from build123d import *

# Parameters (mm, degrees)
SKETCH1_R           = 1.55
SKETCH1_R_2         = 1.6
SKETCH1_W           = 15
SKETCH1_H           = 15
SKETCH1_W_2         = 52
SKETCH1_H_2         = 2.6
BOSS_EXTRUDE1_DEPTH = 2.5
SKETCH2_W           = 144
SKETCH2_H           = 40
BOSS_EXTRUDE2_DEPTH = 2.5


with BuildPart() as part:
    # Sketch1 → Boss-Extrude1 (new body)
    with BuildSketch(Plane(origin=(0, 0, 0), x_dir=(1, 0, 0), z_dir=(0, 1, 0))):
        Polygon((-72, -25), (-76, -25), (-76, 25), (-72, 25), (-72, 72.1), (72, 72.1), (72, 25), (76, 25), (76, -25), (72, -25), (72, -72.1), (-72, -72.1), align=None)
        with Locations((0, -10.804905882)):
            Circle(SKETCH1_R, mode=Mode.SUBTRACT)
        with Locations((0, 9.195094118)):
            Circle(SKETCH1_R, mode=Mode.SUBTRACT)
        with Locations((-49.186770493, 40.239784928)):
            Circle(SKETCH1_R, mode=Mode.SUBTRACT)
        with Locations((49.186770493, 40.239784928)):
            Circle(SKETCH1_R, mode=Mode.SUBTRACT)
        with Locations((-41.500164476, -56.081111214)):
            Circle(SKETCH1_R, mode=Mode.SUBTRACT)
        with Locations((41.500164476, -56.081111214)):
            Circle(SKETCH1_R, mode=Mode.SUBTRACT)
        with Locations((-23, 30.701748775)):
            Circle(SKETCH1_R_2, mode=Mode.SUBTRACT)
        with Locations((24.1, 32.301748775)):
            Circle(SKETCH1_R_2, mode=Mode.SUBTRACT)
        with Locations((23.5, -42.798251225)):
            Circle(SKETCH1_R_2, mode=Mode.SUBTRACT)
        with Locations((-23, -41.598251225)):
            Circle(SKETCH1_R_2, mode=Mode.SUBTRACT)
        with Locations((42.5, 52.1)):
            Circle(SKETCH1_R, mode=Mode.SUBTRACT)
        with Locations((-42.5, 52.1)):
            Circle(SKETCH1_R, mode=Mode.SUBTRACT)
        with Locations((61.5, 56)):
            Rectangle(SKETCH1_W, SKETCH1_H, mode=Mode.SUBTRACT)
        with Locations((-61.5, 56)):
            Rectangle(SKETCH1_W, SKETCH1_H, mode=Mode.SUBTRACT)
        with Locations((0, -67.8)):
            Rectangle(SKETCH1_W_2, SKETCH1_H_2, mode=Mode.SUBTRACT)
        with Locations((0, 67.8)):
            Rectangle(SKETCH1_W_2, SKETCH1_H_2, mode=Mode.SUBTRACT)
        with Locations((-61.5, -56)):
            Rectangle(SKETCH1_W, SKETCH1_H, mode=Mode.SUBTRACT)
        with Locations((61.5, -56)):
            Rectangle(SKETCH1_W, SKETCH1_H, mode=Mode.SUBTRACT)
    extrude(amount=BOSS_EXTRUDE1_DEPTH)

    # Sketch2 → Boss-Extrude2 (add)
    with BuildSketch(Plane(origin=(0, 2.5, 0), x_dir=(1, 0, 0), z_dir=(0, 1, 0))):
        with Locations((0, 92.1)):
            Rectangle(SKETCH2_W, SKETCH2_H)
    extrude(amount=-BOSS_EXTRUDE2_DEPTH)


solid = part.part
Source: CAD feature listing. Evaluate the final solid. Frame: model axes, mm. Give positions to 0.01 mm unless a question says otherwise; leave off trailing zeros. Write each loop counter-clockwise with the first axis right and the second up, starting at its lowest first coordinate (ties: lowest second). Pieces come first, ordered by that corner, then holes. Notation, with made-up numbers: M -19,54.5 L 18,54.5 A31 ccw 18,86.5 Z; hole C 69.5,36.5 d2. An arc over 180 degrees is marked long. Answer as a JSON object with one key per item and string values.
Q1. Cut plane C-C, the plane y = 1. Count the separate pieces of the cut face and the enclosed holes in it, then the cut area to 3 significant figures.
Geometry check:
{"separate pieces": "1", "enclosed holes": "18", "area": "25,700 mm^2"}
Q2. Ray query, line 1 along X through (y, z) = (0.1, 54.5); line 2 along Z through (x, y) = (-59, 1.45); line 3 along Z through (x, y) = (0, 1.75). Return the intervals inside material, ascending.
Geometry check:
{"line 1": "x = -72 to -69, -54 to 54, 69 to 72", "line 2": "z = -112.1 to -63.5, -48.5 to 48.5, 63.5 to 72.1", "line 3": "z = -112.1 to -69.1, -66.5 to -10.75, -7.65 to 9.25, 12.35 to 66.5, 69.1 to 72.1"}
Q3. Cut plane A-A, the plane x = 5.5. Return the cut outline in (y, z), then the cut area to 4 significant figures.
Geometry check:
{"outline": "M 0,-112.1 L 2.5,-112.1 L 2.5,-69.1 L 0,-69.1 Z; M 0,-66.5 L 2.5,-66.5 L 2.5,66.5 L 0,66.5 Z; M 0,69.1 L 2.5,69.1 L 2.5,72.1 L 0,72.1 Z", "area": "447.5 mm^2"}
Q4. Contact query for flat-ended pins moving along their axis: P1, Ø1.9, axis at x = 0, z = 10.8, coming from the +Y side; P2, Ø1.2, axis at y = 1, z = -68, coming from the +X side. Output: stop coordinate, or through.
Geometry check:
{"P1": "passes through", "P2": "stops at x = 72"}
Q5. Cut plane B-B, the plane z = 50.5. Return the cut outline in (x, y).
Geometry check:
{"outline": "M -72,0 L -69,0 L -69,2.5 L -72,2.5 Z; M -54,0 L 54,0 L 54,2.5 L -54,2.5 Z; M 69,0 L 72,0 L 72,2.5 L 69,2.5 Z"}
